Geometry check sheet. Reference: the model listing, model coordinates, mm. A direction names the side the tool comes from. Coordinates: 2 decimals unless noted, no trailing zeros. Write each loop counter-clockwise with the first axis right and the second up, starting at its lowest first coordinate (ties: lowest second). Pieces come first, ordered by that corner, then holes. Notation, with made-up numbers: (55.5, 15.5) -> (103.5, 15.5) arc R34 cw to (103.5, 54.5) -> close; hole circle Ø6 at (16.25, 51.25). An arc over 180 degrees is marked (long way). Use a Markdown table: item, result.
```python
from build123d import *

# Parameters (mm, degrees)
BOSS_EXTRUDE1_DEPTH = 31.75
SKETCH2_W           = 19.05
SKETCH2_H           = 6.35
CUT_EXTRUDE1_DEPTH  = 134.744025007
FILLET1_R           = 5.08
FILLET2_R           = 2.54


with BuildPart() as part:
    # Sketch1 → Boss-Extrude1 (new body)
    with BuildSketch(Plane.XY):
        Polygon((0, 0), (0, 41.275), (123.19, 41.275), (123.19, 0), (120.015, 0), (120.015, 38.1), (3.175, 38.1), (3.175, 0), align=None)
    extrude(amount=BOSS_EXTRUDE1_DEPTH)

    # Sketch2 → Cut-Extrude1 (cut, through all)
    with BuildSketch(Plane.ZY):
        with Locations((15.875, 9.525)):
            Rectangle(SKETCH2_W, SKETCH2_H)
    extrude(amount=-CUT_EXTRUDE1_DEPTH, mode=Mode.SUBTRACT)

    # Fillet1
    fillet1_edges = [part.edges().sort_by_distance(p)[0] for p in [
        (0, 41.275, 15.875),
        (123.19, 41.275, 15.875),
        (120.015, 38.1, 15.875),
        (3.175, 38.1, 15.875),
    ]]
    fillet(fillet1_edges, radius=FILLET1_R)

    # Fillet2
    fillet2_edges = [part.edges().sort_by_distance(p)[0] for p in [
        (120.015, 0, 15.875),
        (3.175, 0, 15.875),
    ]]
    fillet(fillet2_edges, radius=FILLET2_R)


solid = part.part
```
Item 1: Section check C-C on y = 9. Record the boundary of the cut face in (x, z) (3 decimals).
Answer block:
| item | result |
|---|---|
| outline | (0, 0) -> (3.175, 0) -> (3.175, 6.35) -> (0, 6.35) -> close; (0, 25.4) -> (3.175, 25.4) -> (3.175, 31.75) -> (0, 31.75) -> close; (120.015, 0) -> (123.19, 0) -> (123.19, 6.35) -> (120.015, 6.35) -> close; (120.015, 25.4) -> (123.19, 25.4) -> (123.19, 31.75) -> (120.015, 31.75) -> close |
Item 2: Depth check by flat-ended pin: P1, Ø1, axis at x = 2.5, z = 20.5, coming from the -Y side; P2, Ø2.5, axis at x = 1, y = 8, coming from the -Z side; P3, Ø2.5, axis at x = 1, z = 13.5, coming from the +Y side; P4, Ø2.5, axis at x = 121, z = 17, coming from the -Y side. Enter the tip coordinate at first touch or a pass-through.
Answer block:
| item | result |
|---|---|
| P1 | stops at y = 0.4 |
| P2 | stops at z = 0 |
| P3 | stops at y = 40.41 |
| P4 | stops at y = 0.02 |
Item 3: Section check B-B on y = 22.5. Record the boundary of the cut face in (x, z) (3 decimals), then the cut area to 3 significant figures.
Answer block:
| item | result |
|---|---|
| outline | (0, 0) -> (3.175, 0) -> (3.175, 31.75) -> (0, 31.75) -> close; (120.015, 0) -> (123.19, 0) -> (123.19, 31.75) -> (120.015, 31.75) -> close |
| area | 202 mm^2 |
Item 4: Tool access check on faces 4 (the flat face through (2, 12.7, 16)), 5 (the flat face through (61, 41.275, 16)), 6 (the flat face through (120.015, 18, 16)). Record the directions out of +Z, -Z, +X, -X, +Y, -Y that give a thin tool (end or side, any length) a straight path to the whole face; none if there is none.
Answer block:
| item | result |
|---|---|
| face 4 | +X, -X |
| face 5 | +Z, -Z, +X, -X, +Y |
| face 6 | +Z, -Z, -Y |
Item 5: Thickness scan on L1, parallel to X at y = 32.5, z = 9.5 (3 decimals); L2, parallel to Y at x = 78, z = 5.5 (3 decimals); L3, parallel to X at y = 35.5, z = 17. Record the ranges inside material, lowest first. Write a range as [from, to].
Answer block:
| item | result |
|---|---|
| L1 | x = [0, 3.175], [120.015, 123.19] |
| L2 | y = [38.1, 41.275] |
| L3 | x = [0, 3.82], [119.37, 123.19] |
Item 6: Section check D-D on x = 58.5. Record the boundary of the cut face in (y, z) (3 decimals).
Answer block:
| item | result |
|---|---|
| outline | (38.1, 0) -> (41.275, 0) -> (41.275, 31.75) -> (38.1, 31.75) -> close |
Item 7: Mould release check, pull along Y, two halves, no side actions. Record for faces 1 (the flat face through (122, 12.7, 16)), 2 (the cylindrical face through (1.45, 39.75, 16.1)), 3 (the flat face through (62, 38.1, 16)): +Y half, -Y half, draft (parallel to the pull), parting line (faces both ways), or undercut.
Answer block:
| item | result |
|---|---|
| face 1 | undercut |
| face 2 | +Y half |
| face 3 | -Y half |
Item 8: Section check A-A on z = 9.5. Record the boundary of the cut face in (x, y) (3 decimals), then the cut area to 3 significant figures.
Answer block:
| item | result |
|---|---|
| outline | (0, 0) -> (0.635, 0) arc R2.54 ccw to (3.175, 2.54) -> (3.175, 6.35) -> (0, 6.35) -> close; (0, 12.7) -> (3.175, 12.7) -> (3.175, 33.02) arc R5.08 cw to (8.255, 38.1) -> (114.935, 38.1) arc R5.08 cw to (120.015, 33.02) -> (120.015, 12.7) -> (123.19, 12.7) -> (123.19, 36.195) arc R5.08 ccw to (118.11, 41.275) -> (5.08, 41.275) arc R5.08 ccw to (0, 36.195) -> close; (120.015, 2.54) arc R2.54 ccw to (122.555, 0) -> (123.19, 0) -> (123.19, 6.35) -> (120.015, 6.35) -> close |
| area | 590 mm^2 |
